from build123d import *

# Parameters (mm, degrees)
BASE_DEPTH              = 3
ESQUISSE2_W             = 20
ESQUISSE2_H             = 20
ENL_V_MAT_EXTRU_1_DEPTH = 4
CONG_1_R                = 3
ESQUISSE4_R             = 1.25
ESQUISSE4_R_2           = 1.5
ENL_V_MAT_EXTRU_4_DEPTH = 4
ENL_V_MAT_EXTRU_5_REACH = 5
ESQUISSE5_R             = 2.25
ESQUISSE5_W             = 15.031140496
ESQUISSE5_H             = 52.322618027
PONT_H_MAL_PLACE_2_R    = 1.75
PONT_H_MAL_PLACE_DEPTH  = 3
ESQUISSE10_W            = 10
ESQUISSE10_H            = 3
ESQUISSE10_W_2          = 3
ESQUISSE10_H_2          = 30
ENL_V_MAT_EXTRU_7_DEPTH = 3


with BuildPart() as part:
    # Esquisse1 → Base (new body)
    with BuildSketch(Plane.XY):
        Polygon((0, 0), (-175, 0), (-199.748737342, 24.748737342), (-199.748737342, 244.748737342), (-175, 269.497474683), (0, 269.497474683), (24.748737342, 244.748737342), (24.748737342, 24.748737342), align=None)
    extrude(amount=BASE_DEPTH)

    # Esquisse2 → Enlèv. mat.-Extru.1 (cut, through all)
    with BuildSketch(Plane.XY.offset(3)):
        with Locations((-142, 256.997474683)):
            Rectangle(ESQUISSE2_W, ESQUISSE2_H)
        with Locations((-142, 12.5)):
            Rectangle(ESQUISSE2_W, ESQUISSE2_H)
        with Locations((-33, 12.5)):
            Rectangle(ESQUISSE2_W, ESQUISSE2_H)
        with Locations((-33, 256.997474683)):
            Rectangle(ESQUISSE2_W, ESQUISSE2_H)
    extrude(amount=-ENL_V_MAT_EXTRU_1_DEPTH, mode=Mode.SUBTRACT)

    # Congé1
    cong_1_edges = [part.edges().sort_by_distance(p)[0] for p in [
        (0, 0, 1.5),
        (-175, 0, 1.5),
        (-199.748737342, 24.748737342, 1.5),
        (-199.748737342, 244.748737342, 1.5),
        (-175, 269.497474683, 1.5),
        (0, 269.497474683, 1.5),
        (24.748737342, 244.748737342, 1.5),
        (24.748737342, 24.748737342, 1.5),
    ]]
    fillet(cong_1_edges, radius=CONG_1_R)

    # Esquisse4 → Enlèv. mat.-Extru.4 (cut, through all)
    with BuildSketch(Plane.XY.offset(3)):
        with Locations((-78.748737342, 98.497474683)):
            Circle(ESQUISSE4_R)
        with Locations((-127.748737342, 98.497474683)):
            Circle(ESQUISSE4_R)
        with Locations((-78.748737342, 40.497474683)):
            Circle(ESQUISSE4_R)
        with Locations((-127.748737342, 40.497474683)):
            Circle(ESQUISSE4_R)
        with Locations((-129.748737342, 185.997474683)):
            Circle(ESQUISSE4_R_2)
        with Locations((-89.248737342, 227.997474683)):
            Circle(ESQUISSE4_R_2)
        with BuildLine():
            Line((-82.748737342, 166.997474683), (-132.748737342, 166.997474683))
            ThreePointArc((-132.748737342, 166.997474683), (-134.162950904, 166.411688245), (-134.748737342, 164.997474683))
            Line((-134.748737342, 164.997474683), (-134.748737342, 148.997474683))
            ThreePointArc((-134.748737342, 148.997474683), (-134.162950904, 147.583261121), (-132.748737342, 146.997474683))
            Line((-132.748737342, 146.997474683), (-82.748737342, 146.997474683))
            ThreePointArc((-82.748737342, 146.997474683), (-81.334523779, 147.583261121), (-80.748737342, 148.997474683))
            Line((-80.748737342, 148.997474683), (-80.748737342, 164.997474683))
            ThreePointArc((-80.748737342, 164.997474683), (-81.334523779, 166.411688245), (-82.748737342, 166.997474683))
        make_face()
    extrude(amount=-ENL_V_MAT_EXTRU_4_DEPTH, mode=Mode.SUBTRACT)

    # Esquisse5 → Enlèv. mat.-Extru.5 (cut, up to next)
    with BuildSketch(Plane.XY.offset(3), mode=Mode.PRIVATE) as enl_v_mat_extru_5_sk1:
        with Locations((-111.738429941, 3.832493236)):
            Circle(ESQUISSE5_R)
    enl_v_mat_extru_5_tool1 = extrude(enl_v_mat_extru_5_sk1.sketch, amount=-ENL_V_MAT_EXTRU_5_REACH, mode=Mode.PRIVATE) & part.part
    add(enl_v_mat_extru_5_tool1.solids().sort_by_distance((-111.73843, 3.832493, 3))[0], mode=Mode.SUBTRACT)
    # Esquisse5 → Enlèv. mat.-Extru.5 (cut, up to next)
    with BuildSketch(Plane.XY.offset(3), mode=Mode.PRIVATE) as enl_v_mat_extru_5_sk2:
        with Locations((-89.268885084, 3.53845203)):
            Circle(ESQUISSE5_R)
    enl_v_mat_extru_5_tool2 = extrude(enl_v_mat_extru_5_sk2.sketch, amount=-ENL_V_MAT_EXTRU_5_REACH, mode=Mode.PRIVATE) & part.part
    add(enl_v_mat_extru_5_tool2.solids().sort_by_distance((-89.268885, 3.538452, 3))[0], mode=Mode.SUBTRACT)
    # Esquisse5 → Enlèv. mat.-Extru.5 (cut, up to next)
    with BuildSketch(Plane.XY.offset(3), mode=Mode.PRIVATE) as enl_v_mat_extru_5_sk3:
        with Locations((-89.268885084, 33.46154797)):
            Circle(ESQUISSE5_R)
    enl_v_mat_extru_5_tool3 = extrude(enl_v_mat_extru_5_sk3.sketch, amount=-ENL_V_MAT_EXTRU_5_REACH, mode=Mode.PRIVATE) & part.part
    add(enl_v_mat_extru_5_tool3.solids().sort_by_distance((-89.268885, 33.461548, 3))[0], mode=Mode.SUBTRACT)
    # Esquisse5 → Enlèv. mat.-Extru.5 (cut, up to next)
    with BuildSketch(Plane.XY.offset(3), mode=Mode.PRIVATE) as enl_v_mat_extru_5_sk4:
        with Locations((-111.738429941, 33.167506764)):
            Circle(ESQUISSE5_R)
    enl_v_mat_extru_5_tool4 = extrude(enl_v_mat_extru_5_sk4.sketch, amount=-ENL_V_MAT_EXTRU_5_REACH, mode=Mode.PRIVATE) & part.part
    add(enl_v_mat_extru_5_tool4.solids().sort_by_distance((-111.73843, 33.167507, 3))[0], mode=Mode.SUBTRACT)
    # Esquisse5 → Enlèv. mat.-Extru.5 (cut, up to next)
    with BuildSketch(Plane.XY.offset(3), mode=Mode.PRIVATE) as enl_v_mat_extru_5_sk5:
        with Locations((-49.05, 12.640927164)):
            Circle(ESQUISSE5_R)
    enl_v_mat_extru_5_tool5 = extrude(enl_v_mat_extru_5_sk5.sketch, amount=-ENL_V_MAT_EXTRU_5_REACH, mode=Mode.PRIVATE) & part.part
    add(enl_v_mat_extru_5_tool5.solids().sort_by_distance((-49.05, 12.640927, 3))[0], mode=Mode.SUBTRACT)
    # Esquisse5 → Enlèv. mat.-Extru.5 (cut, up to next)
    with BuildSketch(Plane.XY.offset(3), mode=Mode.PRIVATE) as enl_v_mat_extru_5_sk6:
        with Locations((-13.95, 9.5)):
            Circle(ESQUISSE5_R)
    enl_v_mat_extru_5_tool6 = extrude(enl_v_mat_extru_5_sk6.sketch, amount=-ENL_V_MAT_EXTRU_5_REACH, mode=Mode.PRIVATE) & part.part
    add(enl_v_mat_extru_5_tool6.solids().sort_by_distance((-13.95, 9.5, 3))[0], mode=Mode.SUBTRACT)
    # Esquisse5 → Enlèv. mat.-Extru.5 (cut, up to next)
    with BuildSketch(Plane.XY.offset(3), mode=Mode.PRIVATE) as enl_v_mat_extru_5_sk7:
        with Locations((-49.05, 59.140927164)):
            Circle(ESQUISSE5_R)
    enl_v_mat_extru_5_tool7 = extrude(enl_v_mat_extru_5_sk7.sketch, amount=-ENL_V_MAT_EXTRU_5_REACH, mode=Mode.PRIVATE) & part.part
    add(enl_v_mat_extru_5_tool7.solids().sort_by_distance((-49.05, 59.140927, 3))[0], mode=Mode.SUBTRACT)
    # Esquisse5 → Enlèv. mat.-Extru.5 (cut, up to next)
    with BuildSketch(Plane.XY.offset(3), mode=Mode.PRIVATE) as enl_v_mat_extru_5_sk8:
        with Locations((-13.95, 61.981854328)):
            Circle(ESQUISSE5_R)
    enl_v_mat_extru_5_tool8 = extrude(enl_v_mat_extru_5_sk8.sketch, amount=-ENL_V_MAT_EXTRU_5_REACH, mode=Mode.PRIVATE) & part.part
    add(enl_v_mat_extru_5_tool8.solids().sort_by_distance((-13.95, 61.981854, 3))[0], mode=Mode.SUBTRACT)
    # Esquisse5 → Enlèv. mat.-Extru.5 (cut, up to next)
    with BuildSketch(Plane.XY.offset(3), mode=Mode.PRIVATE) as enl_v_mat_extru_5_sk9:
        with Locations((8.748737342, 161.897474683)):
            Circle(ESQUISSE5_R)
    enl_v_mat_extru_5_tool9 = extrude(enl_v_mat_extru_5_sk9.sketch, amount=-ENL_V_MAT_EXTRU_5_REACH, mode=Mode.PRIVATE) & part.part
    add(enl_v_mat_extru_5_tool9.solids().sort_by_distance((8.748737, 161.897475, 3))[0], mode=Mode.SUBTRACT)
    # Esquisse5 → Enlèv. mat.-Extru.5 (cut, up to next)
    with BuildSketch(Plane.XY.offset(3), mode=Mode.PRIVATE) as enl_v_mat_extru_5_sk10:
        with Locations((11.889664506, 196.997474683)):
            Circle(ESQUISSE5_R)
    enl_v_mat_extru_5_tool10 = extrude(enl_v_mat_extru_5_sk10.sketch, amount=-ENL_V_MAT_EXTRU_5_REACH, mode=Mode.PRIVATE) & part.part
    add(enl_v_mat_extru_5_tool10.solids().sort_by_distance((11.889665, 196.997475, 3))[0], mode=Mode.SUBTRACT)
    # Esquisse5 → Enlèv. mat.-Extru.5 (cut, up to next)
    with BuildSketch(Plane.XY.offset(3), mode=Mode.PRIVATE) as enl_v_mat_extru_5_sk11:
        with Locations((-37.751262658, 161.897474683)):
            Circle(ESQUISSE5_R)
    enl_v_mat_extru_5_tool11 = extrude(enl_v_mat_extru_5_sk11.sketch, amount=-ENL_V_MAT_EXTRU_5_REACH, mode=Mode.PRIVATE) & part.part
    add(enl_v_mat_extru_5_tool11.solids().sort_by_distance((-37.751263, 161.897475, 3))[0], mode=Mode.SUBTRACT)
    # Esquisse5 → Enlèv. mat.-Extru.5 (cut, up to next)
    with BuildSketch(Plane.XY.offset(3), mode=Mode.PRIVATE) as enl_v_mat_extru_5_sk12:
        with Locations((-40.592189823, 196.997474683)):
            Circle(ESQUISSE5_R)
    enl_v_mat_extru_5_tool12 = extrude(enl_v_mat_extru_5_sk12.sketch, amount=-ENL_V_MAT_EXTRU_5_REACH, mode=Mode.PRIVATE) & part.part
    add(enl_v_mat_extru_5_tool12.solids().sort_by_distance((-40.59219, 196.997475, 3))[0], mode=Mode.SUBTRACT)
    # Esquisse5 → Enlèv. mat.-Extru.5 (cut, up to next)
    with BuildSketch(Plane.XY.offset(3), mode=Mode.PRIVATE) as enl_v_mat_extru_5_sk13:
        with Locations((-18.655958793, 109.451399186)):
            Circle(ESQUISSE5_R)
    enl_v_mat_extru_5_tool13 = extrude(enl_v_mat_extru_5_sk13.sketch, amount=-ENL_V_MAT_EXTRU_5_REACH, mode=Mode.PRIVATE) & part.part
    add(enl_v_mat_extru_5_tool13.solids().sort_by_distance((-18.655959, 109.451399, 3))[0], mode=Mode.SUBTRACT)
    # Esquisse5 → Enlèv. mat.-Extru.5 (cut, up to next)
    with BuildSketch(Plane.XY.offset(3), mode=Mode.PRIVATE) as enl_v_mat_extru_5_sk14:
        with Locations((-18.95, 86.981854328)):
            Circle(ESQUISSE5_R)
    enl_v_mat_extru_5_tool14 = extrude(enl_v_mat_extru_5_sk14.sketch, amount=-ENL_V_MAT_EXTRU_5_REACH, mode=Mode.PRIVATE) & part.part
    add(enl_v_mat_extru_5_tool14.solids().sort_by_distance((-18.95, 86.981854, 3))[0], mode=Mode.SUBTRACT)
    # Esquisse5 → Enlèv. mat.-Extru.5 (cut, up to next)
    with BuildSketch(Plane.XY.offset(3), mode=Mode.PRIVATE) as enl_v_mat_extru_5_sk15:
        with Locations((10.973095941, 86.981854328)):
            Circle(ESQUISSE5_R)
    enl_v_mat_extru_5_tool15 = extrude(enl_v_mat_extru_5_sk15.sketch, amount=-ENL_V_MAT_EXTRU_5_REACH, mode=Mode.PRIVATE) & part.part
    add(enl_v_mat_extru_5_tool15.solids().sort_by_distance((10.973096, 86.981854, 3))[0], mode=Mode.SUBTRACT)
    # Esquisse5 → Enlèv. mat.-Extru.5 (cut, up to next)
    with BuildSketch(Plane.XY.offset(3), mode=Mode.PRIVATE) as enl_v_mat_extru_5_sk16:
        with Locations((10.679054734, 109.451399186)):
            Circle(ESQUISSE5_R)
    enl_v_mat_extru_5_tool16 = extrude(enl_v_mat_extru_5_sk16.sketch, amount=-ENL_V_MAT_EXTRU_5_REACH, mode=Mode.PRIVATE) & part.part
    add(enl_v_mat_extru_5_tool16.solids().sort_by_distance((10.679055, 109.451399, 3))[0], mode=Mode.SUBTRACT)
    # Esquisse5 → Enlèv. mat.-Extru.5 (cut, up to next)
    with BuildSketch(Plane.XY.offset(3), mode=Mode.PRIVATE) as enl_v_mat_extru_5_sk17:
        with Locations((-60.577832016, 26.161309014)):
            Rectangle(ESQUISSE5_W, ESQUISSE5_H)
    enl_v_mat_extru_5_tool17 = extrude(enl_v_mat_extru_5_sk17.sketch, amount=-ENL_V_MAT_EXTRU_5_REACH, mode=Mode.PRIVATE) & part.part
    add(enl_v_mat_extru_5_tool17.solids().sort_by_distance((-60.577832, 26.161309, 3))[0], mode=Mode.SUBTRACT)

    # PONT H mal place 2 → pont_H_mal_place (cut)
    with BuildSketch(Plane.XY.offset(3)):
        with Locations((-69.262539319, 120.947398703)):
            Circle(PONT_H_MAL_PLACE_2_R)
        with Locations((-69.262539319, 84.205598383)):
            Circle(PONT_H_MAL_PLACE_2_R)
        with Locations((-31.776164099, 84.205598383)):
            Circle(PONT_H_MAL_PLACE_2_R)
        with Locations((-31.776164099, 120.947398703)):
            Circle(PONT_H_MAL_PLACE_2_R)
    extrude(amount=-PONT_H_MAL_PLACE_DEPTH, mode=Mode.SUBTRACT)

    # Esquisse10 → Enlèv. mat.-Extru.7 (cut)
    with BuildSketch(Plane.XY.offset(3)):
        with Locations((-176.748737342, 58.248737342)):
            Rectangle(ESQUISSE10_W, ESQUISSE10_H)
        with Locations((-188.248737342, 95.748737342)):
            Rectangle(ESQUISSE10_W_2, ESQUISSE10_H_2)
        with Locations((-156.748737342, 58.248737342)):
            Rectangle(ESQUISSE10_W, ESQUISSE10_H)
        with Locations((-145.248737342, 95.748737342)):
            Rectangle(ESQUISSE10_W_2, ESQUISSE10_H_2)
        with Locations((-188.248737342, 173.748737342)):
            Rectangle(ESQUISSE10_W_2, ESQUISSE10_H_2)
        with Locations((-156.748737342, 211.248737342)):
            Rectangle(ESQUISSE10_W, ESQUISSE10_H)
        with Locations((-176.748737342, 211.248737342)):
            Rectangle(ESQUISSE10_W, ESQUISSE10_H)
        with Locations((-145.248737342, 173.748737342)):
            Rectangle(ESQUISSE10_W_2, ESQUISSE10_H_2)
    extrude(amount=-ENL_V_MAT_EXTRU_7_DEPTH, mode=Mode.SUBTRACT)


solid = part.part
Work out the finished part from the listing and answer in its coordinate system (mm). Round coordinates to 2 decimals unless told otherwise and drop trailing zeros. Write each loop counter-clockwise with the first axis right and the second up, starting at its lowest first coordinate (ties: lowest second). Pieces come first, ordered by that corner, then holes. Notation, with made-up numbers: (14, 72) - (20, 72) arc R34 cw to (20, 105) - close; hole circle Ø11 at (34, 4). An arc over 180 degrees is marked (long way). Answer in a Markdown table with one row per item. Add a question column.
1. Given pin 1 (3.5 mm diameter, centred on x = -89.27, y = 33.46, fed in from +Z); pin 2 (1.5 mm diameter, centred on y = 8.5, z = 2, fed in from -X); pin 3 (6 mm diameter, centred on x = 8.75, y = 161.9, fed in from -Z), each flat-ended and moving along its own axis, determine where each tip first touches the part or whether it passes through.
2. A cutting plane is placed at B-B, the plane z = 2.15. Count the separate pieces of the cut face and the enclosed holes in it, and give its area (3 significant figures).
3. Find the intervals of material crossed by line 1 along Y through (x, z) = (-49.05, 1.4); line 2 along X through (y, z) = (172, 0.5); line 3 along Y through (x, z) = (-13.95, 0.6), in increasing order. Write a range as from..to.
4. A cutting plane is placed at A-A, the plane y = 153. Determine the outline of the cut face in (x, z).
Worked out:
| question | item | result |
|---|---|---|
| 1 | pin 1 | through |
| 1 | pin 2 | x = -184.25 |
| 1 | pin 3 | z = 0 |
| 2 | separate pieces | 1 |
| 2 | enclosed holes | 39 |
| 2 | area | 55,000 mm^2 |
| 3 | line 1 | 0..10.39, 14.89..56.89, 61.39..269.5 |
| 3 | line 2 | -199.75..-189.75, -186.75..-146.75, -143.75..24.75 |
| 3 | line 3 | 0..7.25, 11.75..59.73, 64.23..269.5 |
| 4 | outline | (-199.75, 0) - (-134.75, 0) - (-134.75, 3) - (-199.75, 3) - close; (-80.75, 0) - (24.75, 0) - (24.75, 3) - (-80.75, 3) - close |
